Geometry check sheet. Reference: drawing and pictorial views, mm from the part's lowest x, y, z. A direction names the side the tool comes from. Coordinates: 2 decimals unless noted, no trailing zeros. Loops run counter-clockwise (first coordinate to the right, second up) from the corner with the lowest first, then second, coordinate; pieces in that order, holes last. Notation, with made-up numbers: (-15.75, 68.25) -> (25.25, 68.25) arc R17 ccw to (25.25, 76.25) -> close; hole circle Ø8 at (-8, -32). An arc over 180 degrees is marked (long way). Answer as a JSON object with one key per item and string values. Group by question number.
Q1. Cross-section at A-A on y = 9. Record the boundary of the cut face in (x, z), and give its area (3 significant figures).
Q2. Cross-section at C-C on z = 3. Record the boundary of the cut face in (x, y), and give its area (3 significant figures).
Q3. Set-up check for the marked faces 1 and 2: record each of +Z, -Z, +X, -X, +Y, -Y from which the full face is reachable in a straight line by a thin tool's end or side.
Q4. Scan lines: L1, parallel to X at y = 1.9, z = 3; L2, parallel to Y at x = 1.8, z = 3; L3, parallel to X at y = 1.5, z = 4.1. Record each from-to range of solid material in increasing order.
Q5. Gauge pin test, flat end, axial feed: pin 1 Ø1 at (y, z) = (5.5, 5.5) entering from +X. Record the tip position at first contact, or that the pin passes through.
Q6. Release check for a two-part mould opening along Z. For the marked faces 3, 4 and 5 record: released by +Z, released by -Z, zero draft, split by the parting line, or undercut.
Q7. Cross-section at D-D on y = 2.5. Record the boundary of the cut face in (x, z).
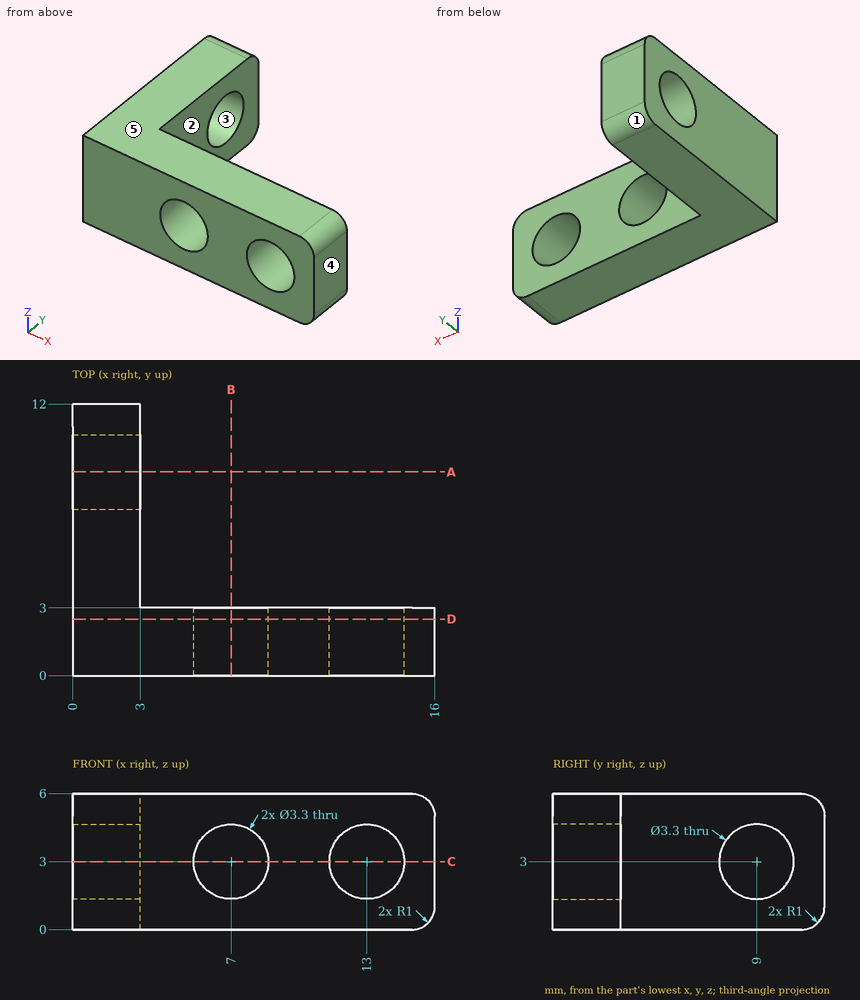
Computed values:
{
 "1": {"outline": "(0, 0) -> (3, 0) -> (3, 1.35) -> (0, 1.35) -> close; (0, 4.65) -> (3, 4.65) -> (3, 6) -> (0, 6) -> close", "area": "8.10 mm²"},
 "2": {"outline": "(0, 0) -> (5.35, 0) -> (5.35, 3) -> (3, 3) -> (3, 7.35) -> (0, 7.35) -> close; (0, 10.65) -> (3, 10.65) -> (3, 12) -> (0, 12) -> close; (8.65, 0) -> (11.35, 0) -> (11.35, 3) -> (8.65, 3) -> close; (14.65, 0) -> (16, 0) -> (16, 3) -> (14.65, 3) -> close", "area": "45.3 mm²"},
 "3": {"face 1": "-Z, +X, -X, +Y", "face 2": "+Z, -Z, +X, +Y"},
 "4": {"L1": "x = 0 to 5.35, 8.65 to 11.35, 14.65 to 16", "L2": "y = 0 to 7.35, 10.65 to 12", "L3": "x = 0 to 5.77, 8.23 to 11.77, 14.23 to 16"},
 "5": {"pin 1": "stops at x = 3"},
 "6": {"face 3": "undercut", "face 4": "zero draft", "face 5": "released by +Z"},
 "7": {"outline": "(0, 0) -> (15, 0) arc R1 ccw to (16, 1) -> (16, 5) arc R1 ccw to (15, 6) -> (0, 6) -> close; hole circle Ø3.3 at (7, 3); hole circle Ø3.3 at (13, 3)"}
}
